Autodesk Inventor part; units mm, degrees
ref_plane "YZ Plane" through (0, 0, 0) normal (1, 0, 0) x (0, 1, 0)
ref_plane "XZ Plane" through (0, 0, 0) normal (0, 1, 0) x (-1, 0, 0)
ref_plane "XY Plane" through (0, 0, 0) normal (0, 0, 1) x (1, 0, 0)
sketch "スケッチ1" plane through (0, 0, 0) normal (0, 1, 0) x (-1, 0, 0)
  line L0 (0, 0) -> (15, 0)
  line L1 (15, 0) -> (15, -50)
  line L2 (15, -50) -> (0, -50)
  line L3 (0, -50) -> (0, 0)
  circle A0 centre (7.5, -8) radius 1.75
  circle A1 centre (7.5, -23) radius 1.75
  dimension "d0" = 15
  dimension "d1" = 50
  dimension "d2" = 15
  dimension "d3" = 3.5
  dimension "d4" = 3.5
  dimension "d5" = 0
  dimension "d6" = 7.5
  dimension "d7" = 8
extrude "押し出し1" add sketch "スケッチ1" along normal blind 6
sketch "スケッチ2" plane through (0, 6, 0) normal (0, 1, 0) x (1, 0, 0)
  line L0 (0, 0) -> (0, 50)
  line L1 (0, 50) -> (-15, 50)
  line L2 (-15, 50) -> (0, 50)
  line L3 (0, 50) -> (0, 42)
  line L4 (0, 42) -> (-15, 42)
  line L5 (-15, 42) -> (-15, 50)
  dimension "d10" = 8
extrude "押し出し2" add sketch "スケッチ2" along normal blind 20.5
sketch "スケッチ3" plane through (0, 26.5, 0) normal (0, 1, 0) x (1, 0, 0)
  line L0 (-15, 50) -> (-15, 42)
  line L1 (0, 42) -> (-44, 42)
  line L2 (-44, 42) -> (-44, 50)
  line L3 (-44, 50) -> (0, 50)
  line L4 (0, 50) -> (0, 42)
  point P0 (0, 0)
  dimension "d13" = 29
  dimension "d14" = 8
extrude "押し出し3" add sketch "スケッチ3" along normal blind 10
sketch "スケッチ4" plane through (-44, 26.5, -50) normal (-1, 0, 0) x (0, 0, 1)
  line L0 (50, -26.5) -> (0, -26.5)
  line L1 (50, -26.5) -> (50, -20.5)
  line L2 (8, -20.5) -> (50, -20.5)
  line L3 (8, -20.5) -> (8, 0)
  line L4 (0, 0) -> (8, 0)
  line L5 (0, -26.5) -> (0, 0)
  line L6 (8, 10) -> (0, 10)
  line L7 (0, 10) -> (0, -26.5)
  line L8 (0, -26.5) -> (8, -26.5)
  line L9 (8, -26.5) -> (8, 10)
  point P0 (50, -26.5)
extrude "押し出し4" add sketch "スケッチ4" along normal blind 10 contours L0 L5 L4 L3 L9 | L7 L6 L9 L4
fillet "フィレット1" radius 6 1 edges at (-44, 0, -46)
fillet "フィレット2" radius 2 23 edges at (-44, 16.25, -42) (-52, 0, -42) (-29.5, 26.5, -42) (-15, 16.25, -42) (0, 18.25, -50) (-27, 36.5, -50) (-54, 18.25, -42) (-54, 18.25, -50) (-54, 0, -46) (-44, 16.25, -50) (-52, 0, -50) (-15, 6, -21) (-7.5, 6, 0) (0, 6, -21) (0, 3, 0) (-15, 13.25, -50) (0, 21.25, -42) (-27, 36.5, -42) (-15, 3, 0) (-29.5, 26.5, -50) (-7.5, 0, -50) (-15, 0, -25) (0, 0, -25)
sketch "スケッチ5" plane through (0, 6, 0) normal (0, 1, 0) x (1, 0, 0)
  circle A0 centre (-7.5, 8) radius 1.75
  circle A1 centre (-7.5, 23) radius 1.75
  line L0 (-15, 44) -> (-15, 2)
  line L1 (-15, 2) -> (-13, 2)
  line L2 (-13, 2) -> (-13, 42)
  arc A2 (-15, 44) -> (-13, 42) centre (-13, 44) ccw
  line L3 (-2, 42) -> (-2, 2)
  line L4 (-2, 2) -> (0, 2)
  line L5 (0, 2) -> (0, 44)
  arc A3 (-2, 42) -> (0, 44) centre (-2, 44) ccw
  line L6 (-2, 0) -> (-2, 2)
  line L7 (-2, 2) -> (-13, 2)
  line L8 (-13, 2) -> (-13, 0)
  line L9 (-13, 0) -> (-2, 0)
  line L10 (-15, 33.6) -> (0, 33.6)
  line L11 (0, 33.6) -> (0, -0.8351)
  line L12 (0, -0.8351) -> (-15, -0.8351)
  line L13 (-15, -0.8351) -> (-15, 33.6)
  point P0 (0, 0)
  dimension "d21" = 10.6
extrude "押し出し5" cut sketch "スケッチ5" against normal blind 2.5 contours A0 | A1 | L10 L2 L1 L0 | L1 L8 L9 L6 L4 L11 L12 L13 | L10 L3 L7 L2 | L7 L6 L9 L8 | L10 L5 L4 L3
sketch "スケッチ6" plane through (0, 0, 0) normal (0, -1, 0) x (1, 0, 0)
  circle A0 centre (-10.9574, -45.6442) radius 1.4
  circle A1 centre (-3.9574, -45.6442) radius 1.4
  point P0 (0, 0)
  dimension "d24" = 2.8
  dimension "d25" = 2.8
  dimension "d26" = 0
  dimension "d27" = 7
extrude "押し出し6" cut sketch "スケッチ6" against normal blind 15
sketch "スケッチ7" plane through (0, 0, 0) normal (0, -1, 0) x (1, 0, 0)
  circle A0 centre (-10.9574, -45.6442) radius 1.4
  circle A1 centre (-3.9574, -45.6442) radius 1.4
  circle A2 centre (-10.9574, -45.6442) radius 2.4
  circle A3 centre (-3.9574, -45.6442) radius 2.4
  point P0 (0, 0)
  dimension "d30" = 1
  dimension "d31" = 1
extrude "押し出し7" cut sketch "スケッチ7" against normal blind 3
fillet "フィレット3" radius 1 2 edges at (-13.3574, 3, -45.6442) (-6.3574, 3, -45.6442)
sketch "スケッチ8" plane through (0, 0, 0) normal (0, -1, 0) x (1, 0, 0)
  circle A0 centre (-7.5, -23) radius 1.75
  circle A1 centre (-7.5, -8) radius 1.75
  circle A2 centre (-7.5, -8) radius 3.25
  circle A3 centre (-7.5, -23) radius 3.25
  point P0 (0, 0)
  dimension "d35" = 1.5
  dimension "d36" = 1.5
extrude "押し出し8" cut sketch "スケッチ8" against normal blind 1
equation "\"d4\" = d3"
equation "\"d6\" = 0.5 * d0"
equation "\"d25\" = d24"
equation "\"d31\" = d30"
equation "\"d36\" = d35"
properties part number "bed-hook"
Here's how the part is built. I have some questions about the finished solid (model axes, mm). A direction names the side the tool comes from. Give positions to 0.01 mm unless a question says otherwise; leave off trailing zeros. Loops run counter-clockwise (first coordinate to the right, second up) from the corner with the lowest first, then second, coordinate; pieces in that order, holes last. Notation, with made-up numbers: (31, 53) -> (64, 53) arc R14 ccw to (64, 62) -> close; hole circle Ø1 at (-38, -21). An arc over 180 degrees is marked (long way). Answer as a JSON object with one key per item and string values. Group by question number.
Item 1: Imagine slicing it at C-C on x = -7.5. Write out the boundary of the cut face in (y, z), then the cut area to 3 significant figures.
Item 2: Imagine slicing it at D-D on x = -51. Write out the boundary of the cut face in (y, z), then the cut area to 3 significant figures.
Item 3: Will these pins go through, and if not, where does the flat tip stop? pin 1 (3 mm diameter, centred on x = -8, z = -24, fed in from -Y); pin 2 (3 mm diameter, centred on y = 20, z = -47, fed in from +X); pin 3 (0.8 mm diameter, centred on x = -11.5, z = -45.5, fed in from -Y); pin 4 (2 mm diameter, centred on x = -7, y = 28, fed in from +Z).
Item 4: I need wall thicknesses on L1, parallel to Z at x = -7.5, y = 1.9; L2, parallel to X at y = 8, z = -45.5; L3, parallel to Z at x = -7.5, y = 0.2. Which ranges of each line are inside material? Lowest first, please.
Item 5: Thinking about a two-plate mould opening in Z: for faces 1 (the cylindrical face through (-9.169, 2.232, -8.526)), 2 (the cylindrical face through (-14.2, 2.2, -0.4)), 3 (the cylindrical face through (-14.43, 15.06, -49.4)), which applies, pulls with the +Z half, pulls with the -Z half, needs draft (parallel to the pull), parting line crosses it, or undercut?
Item 6: On a 3-axis mill with a long thin cutter (end or side, diameter ignored), from which of +Z, -Z, +X, -X, +Y, -Y can I reach the whole of each face in a straight line? I mean faces 4 (the cylindrical face through (-14.43, 16.42, -42.6)), 5 (the flat face through (-6.1, 1, -9.4)), 6 (the flat face through (-8, 5, -33.6)), 7 (the cylindrical face through (-44.6, 17.09, -49.43)), 8 (the cylindrical face through (-0.87, 2.16, -0.35)). Say none if no direction works.
Item 7: Imagine slicing it at B-B on y = 23. Write out the boundary of the cut face in (x, z), then the cut area to 3 significant figures.
Item 8: Imagine slicing it at A-A on z = -8. Write out the boundary of the cut face in (x, y).
Answer list:
{
 "1": {"outline": "(0, -48) arc R2 ccw to (2, -50) -> (34.5, -50) arc R2 ccw to (36.5, -48) -> (36.5, -44) arc R2 ccw to (34.5, -42) -> (6, -42) -> (6, -33.6) -> (3.5, -33.6) -> (3.5, -24.75) -> (1, -24.75) -> (1, -26.25) -> (0, -26.25) -> close; (0, -19.75) -> (1, -19.75) -> (1, -21.25) -> (3.5, -21.25) -> (3.5, -9.75) -> (1, -9.75) -> (1, -11.25) -> (0, -11.25) -> close; (0, -4.75) -> (1, -4.75) -> (1, -6.25) -> (3.5, -6.25) -> (3.5, 0) -> (0, 0) -> close", "area": "427 mm2"},
 "2": {"outline": "(0, -48) arc R2 ccw to (2, -50) -> (34.5, -50) arc R2 ccw to (36.5, -48) -> (36.5, -44) arc R2 ccw to (34.5, -42) -> (2, -42) arc R2 ccw to (0, -44) -> close", "area": "289 mm2"},
 "3": {"pin 1": "stops at y = 1", "pin 2": "stops at x = 0", "pin 3": "stops at y = 15", "pin 4": "stops at z = -42"},
 "4": {"L1": "z = -50 to -24.75, -21.25 to -9.75, -6.25 to 0", "L2": "x = -54 to -44, -15 to -12.35, -9.56 to -5.35, -2.56 to 0", "L3": "z = -48.87 to -26.25, -19.75 to -11.25, -4.75 to 0"},
 "5": {"face 1": "undercut", "face 2": "pulls with the +Z half", "face 3": "pulls with the -Z half"},
 "6": {"face 4": "+Z", "face 5": "-Y", "face 6": "+Z, +X, -X, +Y", "face 7": "-Z, -Y", "face 8": "+Z, +X, +Y, -Y"},
 "7": {"outline": "(-54, -48) arc R2 ccw to (-52, -50) -> (-46, -50) arc R2 ccw to (-44, -48) -> (-44, -44) arc R2 ccw to (-46, -42) -> (-52, -42) arc R2 ccw to (-54, -44) -> close; (-15, -48) arc R2 ccw to (-13, -50) -> (-2, -50) arc R2 ccw to (0, -48) -> (0, -44) arc R2 ccw to (-2, -42) -> (-13, -42) arc R2 ccw to (-15, -44) -> close", "area": "193 mm2"},
 "8": {"outline": "(-15, 2) arc R2 ccw to (-13, 0) -> (-10.75, 0) -> (-10.75, 1) -> (-9.25, 1) -> (-9.25, 3.5) -> (-15, 3.5) -> close; (-5.75, 1) -> (-4.25, 1) -> (-4.25, 0) -> (-2, 0) arc R2 ccw to (0, 2) -> (0, 3.5) -> (-5.75, 3.5) -> close"}
}
